Answer from the drawing. Dimensions are ordinates in mm from the lowest x, y and z of the part. Coordinates: 2 decimals unless noted, no trailing zeros. Order: outer loops, then holes, each group sorted by start corner. A loop starts at its lowest first (then second) coordinate and runs counter-clockwise, first axis right, second up. Notation, with made-up numbers: M -9,-24.5 L 0,-24.5 A29 cw 0,-0.5 Z; hole C -22,-7.75 d7. An arc over 180 degrees is marked long. Use a Markdown table: item, result.
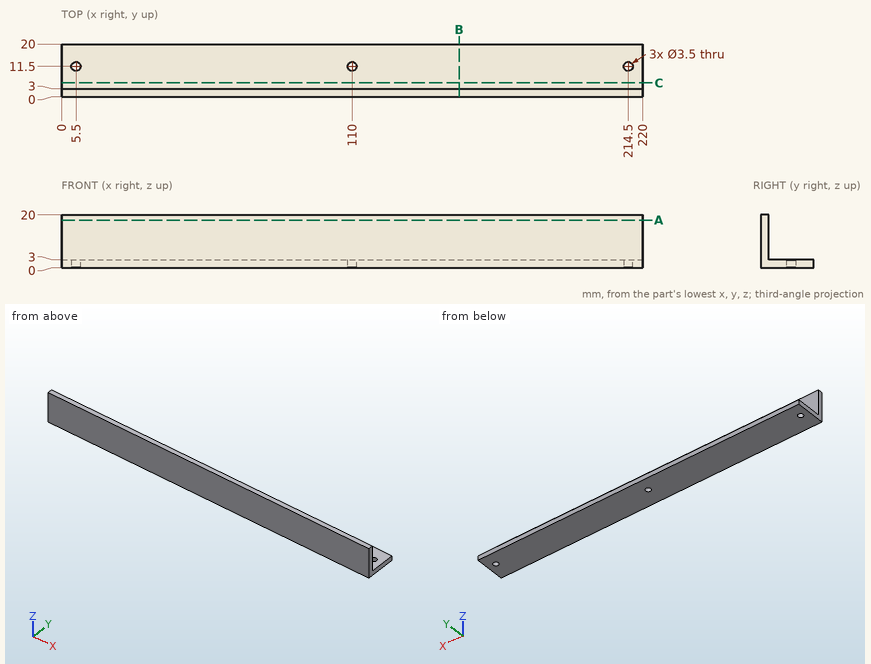
(1) A cutting plane is placed at A-A (z = 18). Determine the outline of the cut face in (x, y).
Conclusion:
| item | result |
|---|---|
| outline | M 0,0 L 220,0 L 220,3 L 0,3 Z |
(2) A cutting plane is placed at B-B (x = 150.5). Determine the outline of the cut face in (y, z), then the cut area to 3 significant figures.
Conclusion:
| item | result |
|---|---|
| outline | M 0,0 L 20,0 L 20,3 L 3,3 L 3,20 L 0,20 Z |
| area | 111 mm2 |
(3) Straight lines are drawn through the part: L1, parallel to X at y = 11.5, z = 2.3; L2, parallel to Y at x = 110, z = 1.05; L3, parallel to Z at x = 33, y = 18.5. For each, find the intervals that lie inside material, in ascending order.
Conclusion:
| item | result |
|---|---|
| L1 | 0 to 3.75, 7.25 to 108.25, 111.75 to 212.75, 216.25 to 220 |
| L2 | 0 to 9.75, 13.25 to 20 |
| L3 | 0 to 3 |
(4) Given P1, Ø1, axis at x = 113, z = 14, coming from the +Y side; P2, Ø3, axis at x = 5.5, y = 11.5, coming from the +Z side; P3, Ø2, axis at x = 182.5, z = 16.5, coming from the -Y side, each flat-ended and moving along its own axis, determine where each tip first touches the part or whether it passes through.
Conclusion:
| item | result |
|---|---|
| P1 | y = 3 |
| P2 | through |
| P3 | y = 0 |
